```python
from build123d import *

# Parameters (mm, degrees)
SKETCH2_R                                          = 3.96875
SKETCH2_R_2                                        = 2.25
BODY_DEPTH                                         = 130
SKETCH4_W                                          = 26.495455659
SKETCH4_H                                          = 4
CAVITY_FOR_SLIDER_DEPTH                            = 4.96875
CAVITY_FOR_SLIDER_DEPTH_BACK                       = 4.96875
SLIDER_TRACK_FOR_M2_SCREW_5_64_END_MILL_DEPTH      = 4.96875
SLIDER_TRACK_FOR_M2_SCREW_5_64_END_MILL_DEPTH_BACK = 4.96875


with BuildPart() as part:
    # Sketch2 → Body (new body)
    with BuildSketch(Plane(origin=(0, 0, 0), x_dir=(0, 0, -1), z_dir=(1, 0, 0))):
        Circle(SKETCH2_R)
        Circle(SKETCH2_R_2, mode=Mode.SUBTRACT)
    extrude(amount=BODY_DEPTH)

    # Sketch4 → cavity for slider (cut, two sides)
    with BuildSketch(Plane(origin=(0, 0, 0), x_dir=(1, 0, 0), z_dir=(0, 1, 0))) as cavity_for_slider_sk:
        with Locations((32.060413051, 0)):
            Rectangle(SKETCH4_W, SKETCH4_H)
    extrude(amount=CAVITY_FOR_SLIDER_DEPTH, mode=Mode.SUBTRACT)
    extrude(cavity_for_slider_sk.sketch, amount=-CAVITY_FOR_SLIDER_DEPTH_BACK, mode=Mode.SUBTRACT)

    # Sketch12 → slider track for M2 screw 5_64 end mill (cut, two sides)
    with BuildSketch(Plane.XY) as slider_track_for_m2_screw_5_64_end_mill_sk:
        with BuildLine():
            Line((39.315953381, -0.9921875), (34.315953381, -0.9921875))
            ThreePointArc((34.315953381, -0.9921875), (33.323765881, 0), (34.315953381, 0.9921875))
            Line((34.315953381, 0.9921875), (39.315953381, 0.9921875))
            ThreePointArc((39.315953381, 0.9921875), (40.308140881, 0), (39.315953381, -0.9921875))
        make_face()
    extrude(amount=SLIDER_TRACK_FOR_M2_SCREW_5_64_END_MILL_DEPTH, mode=Mode.SUBTRACT)
    extrude(slider_track_for_m2_screw_5_64_end_mill_sk.sketch, amount=-SLIDER_TRACK_FOR_M2_SCREW_5_64_END_MILL_DEPTH_BACK, mode=Mode.SUBTRACT)


solid = part.part
```
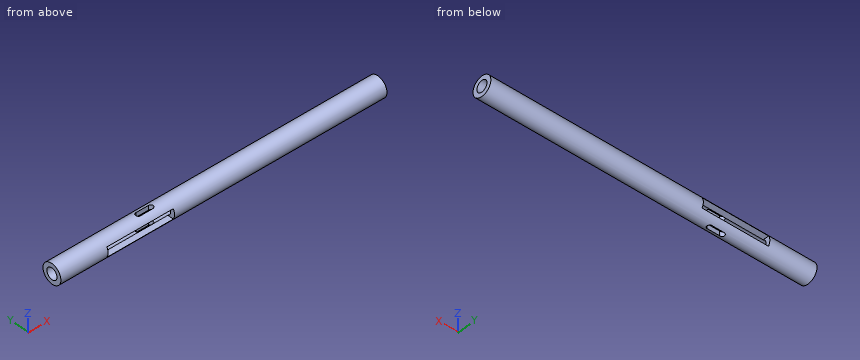
Source: CAD feature listing. Evaluate the final solid. Frame: model axes, mm. Round coordinates to 2 decimals unless told otherwise and drop trailing zeros. Loops run counter-clockwise (first coordinate to the right, second up) from the corner with the lowest first, then second, coordinate; pieces in that order, holes last.
(1) Material intervals for probe 1 along Y at (x, z) = (64.5, 0); probe 2 along X at (y, z) = (2.25, -1.5); probe 3 along Y at (x, z) = (61, 1), sorted ascending.
From the geometry:
probe 1: y = -3.97 to -2.25, 2.25 to 3.97
probe 2: x = 0 to 18.81, 45.31 to 130
probe 3: y = -3.84 to -2.02, 2.02 to 3.84
(2) Section query B-B (x = 54). Output: boundary loops of the cut face in (y, z), and give its area (3 significant figures).
From the geometry:
outline: circle Ø7.94 at (0, 0); hole circle Ø4.5 at (0, 0)
area: 33.6 mm2
(3) Section query A-A (z = 0). Output: boundary loops of the cut face in (x, y).
From the geometry:
outline: (0, -3.97) - (18.81, -3.97) - (18.81, -2.25) - (0, -2.25) - close; (0, 2.25) - (18.81, 2.25) - (18.81, 3.97) - (0, 3.97) - close; (45.31, -3.97) - (130, -3.97) - (130, -2.25) - (45.31, -2.25) - close; (45.31, 2.25) - (130, 2.25) - (130, 3.97) - (45.31, 3.97) - close
(4) Contact query for flat-ended pins moving along their axis: pin 1 Ø2.5 at (x, y) = (37, -2) entering from -Z; pin 2 Ø1.2 at (x, y) = (32.5, 2) entering from +Z; pin 3 Ø2 at (x, z) = (36.5, 2.5) entering from +Y. Output: stop coordinate, or through.
From the geometry:
pin 1: stops at z = -3.84
pin 2: stops at z = 3.71
pin 3: stops at y = 3.43
